Can you work these out from the model? Positions are in its coordinate system, mm. Face numbers are marked on the shaded views. A direction names the side the tool comes from. Coordinates: 2 decimals unless noted, no trailing zeros. Order: outer loops, then holes, each group sorted by start corner. A loop starts at its lowest first (then second) coordinate and runs counter-clockwise, first axis right, second up.
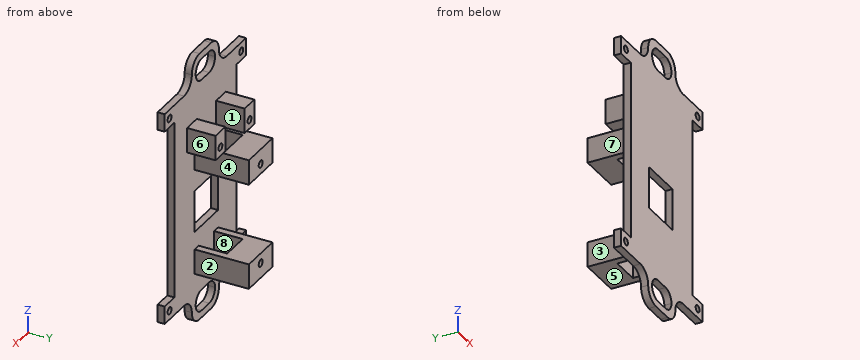
```python
from build123d import *

# Parameters (mm, degrees)
CROQUIS1_R                 = 1
SALIENTE_EXTRUIR2_DEPTH    = 2
SALIENTE_EXTRUIR3_DEPTH    = 15.2
CROQUIS3_R                 = 1
CORTAR_EXTRUIR1_DEPTH      = 8
CROQUIS4_R                 = 1
SALIENTE_EXTRUIR4_DEPTH    = 8
CORTAR_EXTRUIR2_DEPTH      = 51.918821667
CORTAR_EXTRUIR2_DEPTH_BACK = 51.918821667
SALIENTE_EXTRUIR6_DEPTH    = 2
REDONDEO1_R                = 4
CORTAR_EXTRUIR3_DEPTH      = 10


with BuildPart() as part:
    # Croquis1 → Saliente-Extruir2 (new body)
    with BuildSketch(Plane(origin=(0, 0, 0), x_dir=(1, 0, 0), z_dir=(0, 1, 0))):
        Polygon((-21, 30), (-21, 25), (-16, 25), (-16, -25), (-21, -25), (-21, -30), (21, -30), (21, -25), (16, -25), (16, 25), (21, 25), (21, 30), align=None)
        with Locations(Location((-18.5, -27.5, 0), (0, 0, 270))):
            Circle(CROQUIS1_R, mode=Mode.SUBTRACT)
        with Locations(Location((-18.5, 27.5, 0), (0, 0, 270))):
            Circle(CROQUIS1_R, mode=Mode.SUBTRACT)
        with Locations(Location((18.5, 27.5, 0), (0, 0, 270))):
            Circle(CROQUIS1_R, mode=Mode.SUBTRACT)
        with Locations(Location((18.5, -27.5, 0), (0, 0, 270))):
            Circle(CROQUIS1_R, mode=Mode.SUBTRACT)
    extrude(amount=SALIENTE_EXTRUIR2_DEPTH)

    # Croquis2 → Saliente-Extruir3 (add)
    with BuildSketch(Plane(origin=(0, 2, 0), x_dir=(1, 0, 0), z_dir=(0, 1, 0))):
        Polygon((5.549377546, 23.7), (5.549377546, 16.7), (-0.530622454, 16.7), (-6.610622454, 16.7), (-6.610622454, 23.7), align=None)
        Polygon((-6.610622454, -13.08), (5.549377546, -13.08), (5.549377546, -6.08), (-0.530622454, -6.08), (-6.610622454, -6.08), align=None)
    extrude(amount=SALIENTE_EXTRUIR3_DEPTH)

    # Croquis3 → Cortar-Extruir1 (cut)
    with BuildSketch(Plane(origin=(0, 17.2, 0), x_dir=(1, 0, 0), z_dir=(0, 1, 0))):
        with Locations(Location((-0.530622454, 19.48, 0), (0, 0, 270))):
            Circle(CROQUIS3_R)
        with Locations(Location((-0.530622454, -8.86, 0), (0, 0, 270))):
            Circle(CROQUIS3_R)
    extrude(amount=-CORTAR_EXTRUIR1_DEPTH, mode=Mode.SUBTRACT)

    # Croquis4 → Saliente-Extruir4 (add)
    # profile 1 of 2: a face of its own
    with BuildSketch(Plane(origin=(0, 2, 0), x_dir=(1, 0, 0), z_dir=(0, 1, 0))):
        Polygon((-5.530622454, -20.08), (-5.530622454, -13.08), (-6.610622454, -13.08), (-10.530622454, -13.08), (-10.530622454, -20.08), align=None)
        with Locations(Location((-8.030622454, -15.58, 0), (0, 0, 270))):
            Circle(CROQUIS4_R, mode=Mode.SUBTRACT)
    # profile 2 of 2: a face of its own
    with BuildSketch(Plane(origin=(0, 2, 0), x_dir=(1, 0, 0), z_dir=(0, 1, 0))):
        Polygon((9.469377546, -20.08), (9.469377546, -13.08), (5.549377546, -13.08), (4.469377546, -13.08), (4.469377546, -20.08), align=None)
        with Locations(Location((6.969377546, -15.58, 0), (0, 0, 270))):
            Circle(CROQUIS4_R, mode=Mode.SUBTRACT)
    extrude(amount=SALIENTE_EXTRUIR4_DEPTH)

    # Croquis5 → Cortar-Extruir2 (cut, two sides: drawn at the far end of the back side and taken through both)
    with BuildSketch(Plane.XY.offset(13.08).offset(-CORTAR_EXTRUIR2_DEPTH_BACK)):
        Polygon((-4.530622454, 2), (-0.530622454, 2), (3.469377546, 2), (3.469377546, 10), (-4.530622454, 10), align=None)
    extrude(amount=CORTAR_EXTRUIR2_DEPTH + CORTAR_EXTRUIR2_DEPTH_BACK, mode=Mode.SUBTRACT)

    # Croquis6 → Saliente-Extruir6 (add)
    with BuildSketch(Plane(origin=(0, 2, 0), x_dir=(1, 0, 0), z_dir=(0, 1, 0))):
        with BuildLine():
            Line((3.5, 30), (5, 30))
            Line((5, 30), (7, 30))
            Line((7, 30), (7, 34))
            ThreePointArc((7, 34), (5.828427125, 36.828427125), (3, 38))
            Line((3, 38), (-3, 38))
            ThreePointArc((-3, 38), (-5.828427125, 36.828427125), (-7, 34))
            Line((-7, 34), (-7, 30))
            Line((-7, 30), (-5, 30))
            Line((-5, 30), (-3.5, 30))
            Line((-3.5, 30), (-2, 30))
            ThreePointArc((-2, 30), (-4.121320344, 30.878679656), (-5, 33))
            ThreePointArc((-5, 33), (-4.121320344, 35.121320344), (-2, 36))
            Line((-2, 36), (0, 36))
            Line((0, 36), (2, 36))
            ThreePointArc((2, 36), (4.121320344, 35.121320344), (5, 33))
            ThreePointArc((5, 33), (4.121320344, 30.878679656), (2, 30))
            Line((2, 30), (3.5, 30))
        make_face()
        with BuildLine():
            Line((7, -34), (7, -30))
            Line((7, -30), (5, -30))
            Line((5, -30), (3.5, -30))
            Line((3.5, -30), (2, -30))
            ThreePointArc((2, -30), (4.121320344, -30.878679656), (5, -33))
            ThreePointArc((5, -33), (4.121320344, -35.121320344), (2, -36))
            Line((2, -36), (0, -36))
            Line((0, -36), (-2, -36))
            ThreePointArc((-2, -36), (-4.121320344, -35.121320344), (-5, -33))
            ThreePointArc((-5, -33), (-4.121320344, -30.878679656), (-2, -30))
            Line((-2, -30), (-3.5, -30))
            Line((-3.5, -30), (-5, -30))
            Line((-5, -30), (-7, -30))
            Line((-7, -30), (-7, -34))
            ThreePointArc((-7, -34), (-5.828427125, -36.828427125), (-3, -38))
            Line((-3, -38), (3, -38))
            ThreePointArc((3, -38), (5.828427125, -36.828427125), (7, -34))
        make_face()
    extrude(amount=-SALIENTE_EXTRUIR6_DEPTH)

    # Redondeo1
    redondeo1_edges = [part.edges().sort_by_distance(p)[0] for p in [
        (7, 1, -30),
        (-7, 1, -30),
        (-7, 1, 30),
        (7, 1, 30),
    ]]
    fillet(redondeo1_edges, radius=REDONDEO1_R - 0.0001)  # a hair under: the kernel refuses the full size

    # Croquis7 → Cortar-Extruir3 (cut)
    with BuildSketch(Plane(origin=(0, 2, 0), x_dir=(1, 0, 0), z_dir=(0, 1, 0))):
        Polygon((0, 0), (-6.51429836, 0), (-6.51429836, 11.7), (0, 11.7), (5.54570164, 11.7), (5.54570164, 0), align=None)
    extrude(amount=-CORTAR_EXTRUIR3_DEPTH, mode=Mode.SUBTRACT)


solid = part.part
```
1. I'm going to push flat-ended pins straight in: pin 1 (4 mm diameter, centred on x = 8, z = 1, fed in from +Y); pin 2 (1.6 mm diameter, centred on y = 1.5, z = 4.5, fed in from -X); pin 3 (2 mm diameter, centred on y = 4.5, z = 17.5, fed in from +X); pin 4 (8 mm diameter, centred on x = -1.5, y = 5, fed in from -Z). Where does each tip first touch, or does it pass through?
Completed:
pin 1: stops at y = 2
pin 2: stops at x = -16
pin 3: stops at x = 9.47
pin 4: stops at z = -38
2. On a 3-axis mill with a long thin cutter (end or side, diameter ignored), from which of +Z, -Z, +X, -X, +Y, -Y can I reach the whole of each face in a straight line? I mean the marked faces 4, 5, 6, 7 and 8. Say none if no direction works.
Completed:
face 4: -Z, +X, +Y
face 5: -Z, +X, -X, +Y
face 6: +Z, -Z, +X, +Y
face 7: -Z, -X, +Y
face 8: +Z, -Z
3. Thinking about a two-plate mould opening in X: for the marked faces 1, 2 and 3, which applies, pulls with the +X half, pulls with the -X half, needs draft (parallel to the pull), parting line crosses it, or undercut?
Completed:
face 1: undercut
face 2: pulls with the +X half
face 3: pulls with the -X half
4. Imagine slicing it at B-B on z = 27.5. Please give me the cut outline in (x, y), then the cut area to 3 significant figures.
Completed:
outline: (-21, 0) - (-19.5, 0) - (-19.5, 2) - (-21, 2) - close; (-17.5, 0) - (17.5, 0) - (17.5, 2) - (-17.5, 2) - close; (19.5, 0) - (21, 0) - (21, 2) - (19.5, 2) - close
area: 76.0 mm2
5. Imagine slicing it at A-A on y = 12. Please give me the cut outline in (x, z).
Completed:
outline: (-6.61, -23.7) - (5.55, -23.7) - (5.55, -16.7) - (-6.61, -16.7) - close; (-6.61, 6.08) - (5.55, 6.08) - (5.55, 13.08) - (-6.61, 13.08) - close; hole circle Ø2 at (-0.53, -19.48); hole circle Ø2 at (-0.53, 8.86)
6. Please list where these lines run through material, in increasing order: probe 1 along X at (y, z) = (0.7, 27.5); probe 2 along Z at (x, y) = (-5, 4.75); probe 3 along Y at (x, z) = (-3.5, 13).
Completed:
probe 1: x = -21 to -19.5, -17.5 to 17.5, 19.5 to 21
probe 2: z = -23.7 to -16.7, 6.08 to 13.08
probe 3: y = 0 to 2, 10 to 17.2
7. Imagine slicing it at C-C on x = 18.5. Please give me the cut outline in (y, z), then the cut area to 3 significant figures.
Completed:
outline: (0, -30) - (2, -30) - (2, -28.5) - (0, -28.5) - close; (0, -26.5) - (2, -26.5) - (2, -25) - (0, -25) - close; (0, 25) - (2, 25) - (2, 26.5) - (0, 26.5) - close; (0, 28.5) - (2, 28.5) - (2, 30) - (0, 30) - close
area: 12.0 mm2
8. Imagine slicing it at D-D on y = 5. Please give me the cut outline in (x, z).
Completed:
outline: (-10.53, 13.08) - (-6.61, 13.08) - (-6.61, 6.08) - (-4.53, 6.08) - (-4.53, 13.08) - (-5.53, 13.08) - (-5.53, 20.08) - (-10.53, 20.08) - close; (-6.61, -23.7) - (-4.53, -23.7) - (-4.53, -16.7) - (-6.61, -16.7) - close; (3.47, -23.7) - (5.55, -23.7) - (5.55, -16.7) - (3.47, -16.7) - close; (3.47, 6.08) - (5.55, 6.08) - (5.55, 13.08) - (9.47, 13.08) - (9.47, 20.08) - (4.47, 20.08) - (4.47, 13.08) - (3.47, 13.08) - close; hole circle Ø2 at (-8.03, 15.58); hole circle Ø2 at (6.97, 15.58)
